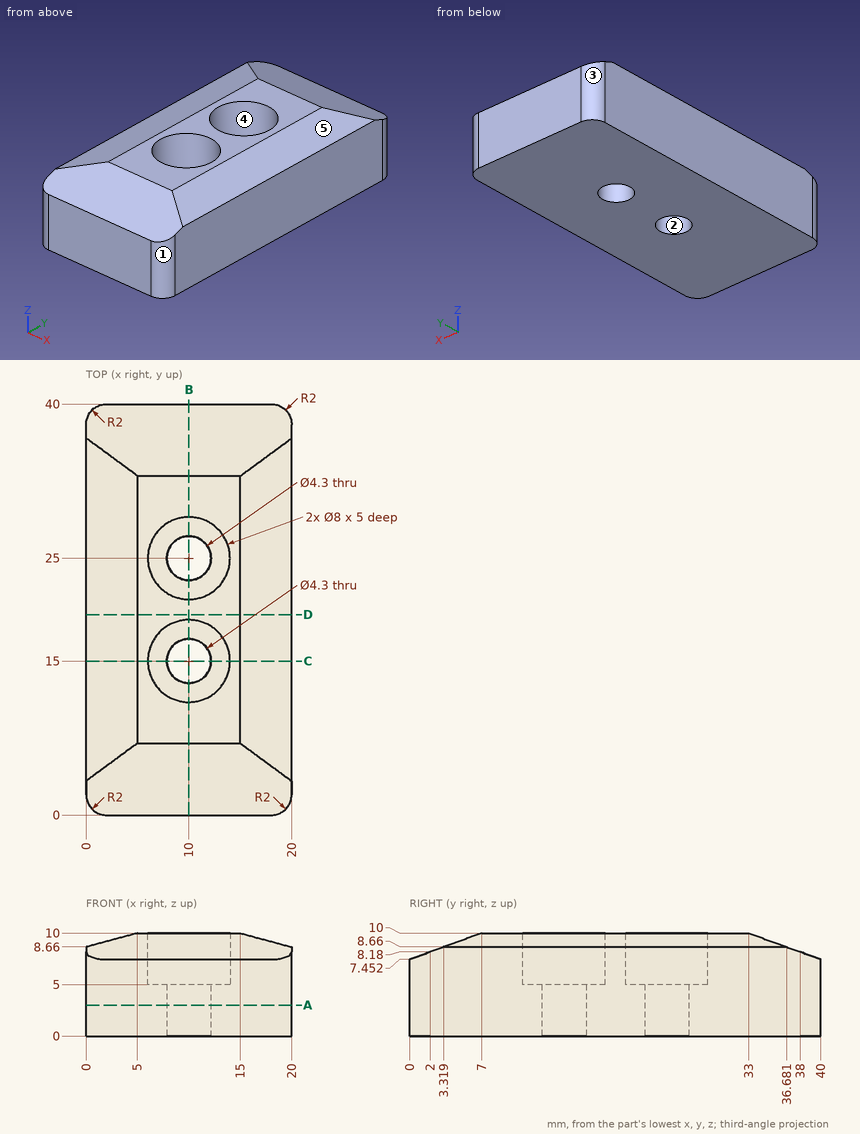
Can you work these out from the drawing? Everything is in mm from the part's minimum corner. A direction names the side the tool comes from. Coordinates: 2 decimals unless noted, no trailing zeros. Order: outer loops, then holes, each group sorted by start corner. A loop starts at its lowest first (then second) coordinate and runs counter-clockwise, first axis right, second up. Notation, with made-up numbers: M 81,-39.75 L 131,-39.75 A32 ccw 131,-4.75 Z; hole C 76,48.25 d3. An arc over 180 degrees is marked long. Answer as CSV lines item,"result". Start each with the question number.
1. For pin 1 (6 mm diameter, centred on x = 16, y = 8.5, fed in from -Z); pin 2 (2.5 mm diameter, centred on x = 9.5, y = 14, fed in from +Z); pin 3 (4 mm diameter, centred on x = 15.5, y = 35, fed in from +Z), each with a flat end and sliding along its axis, tell me the tip position at first contact or that it passes through.
2. We'd pull the mould along Y, two halves only. Please class the marked faces 1, 2 and 3: released by +Y, released by -Y, zero draft, split by the parting line, or undercut.
3. On a 3-axis mill with a long thin cutter (end or side, diameter ignored), from which of +Z, -Z, +X, -X, +Y, -Y can I reach the whole of each face in a straight line? I mean the marked faces 4 and 5. Say none if no direction works.
4. I want a section at C-C, the plane y = 15. Write out the boundary of the cut face in (x, z), and give its area (3 significant figures).
5. I want a section at A-A, the plane z = 3. Write out the boundary of the cut face in (x, y).
6. I want a section at D-D, the plane y = 19.5. Write out the boundary of the cut face in (x, z), and give its area (3 significant figures).
7. I need wall thicknesses on line 1 (Y direction, x = 10, z = 1.85); line 2 (X direction, y = 15, z = 1.2); line 3 (Y direction, x = 13.5, z = 7) (1 decimal). Which ranges of each line are inside material? Lowest first, please. Write a range as [from, to].
8. I want a section at B-B, the plane x = 10. Write out the boundary of the cut face in (y, z).
Recorded:
1,pin 1,"stops at z = 0"
1,pin 2,"stops at z = 5"
1,pin 3,"stops at z = 9.98"
2,face 1,"released by -Y"
2,face 2,"undercut"
2,face 3,"released by +Y"
3,face 4,"+Z"
3,face 5,"+Z, +X, +Y, -Y"
4,outline,"M 0,0 L 7.85,0 L 7.85,5 L 6,5 L 6,10 L 5,10 L 0,8.66 Z; M 12.15,0 L 20,0 L 20,8.66 L 15,10 L 14,10 L 14,5 L 12.15,5 Z"
4,area,"132 mm2"
5,outline,"M 0,2 A2 ccw 2,0 L 18,0 A2 ccw 20,2 L 20,38 A2 ccw 18,40 L 2,40 A2 ccw 0,38 Z; hole C 10,15 d4.3; hole C 10,25 d4.3"
6,outline,"M 0,0 L 20,0 L 20,8.66 L 15,10 L 5,10 L 0,8.66 Z"
6,area,"193 mm2"
7,line 1,"y = [0, 12.85], [17.15, 22.85], [27.15, 40]"
7,line 2,"x = [0, 7.85], [12.15, 20]"
7,line 3,"y = [0, 13.1], [16.9, 23.1], [26.9, 40]"
8,outline,"M 0,0 L 12.85,0 L 12.85,5 L 11,5 L 11,10 L 7,10 L 0,7.45 Z; M 17.15,0 L 22.85,0 L 22.85,5 L 21,5 L 21,10 L 19,10 L 19,5 L 17.15,5 Z; M 27.15,0 L 40,0 L 40,7.45 L 33,10 L 29,10 L 29,5 L 27.15,5 Z"
